Autodesk Inventor part; units mm, degrees
ref_plane "YZ Plane" through (0, 0, 0) normal (1, 0, 0) x (0, 1, 0)
ref_plane "XZ Plane" through (0, 0, 0) normal (0, 1, 0) x (-1, 0, 0)
ref_plane "XY Plane" through (0, 0, 0) normal (0, 0, 1) x (1, 0, 0)
sketch "스케치1" plane through (0, 0, 0) normal (0, 0, 1) x (1, 0, 0)
  line L0 (0, 0) -> (25, 0)
  line L1 (25, 0) -> (25, 16.5)
  line L2 (25, 16.5) -> (0, 16.5)
  line L3 (0, 16.5) -> (0, 0)
  circle A0 centre (23, 14.5) radius 1
  circle A1 centre (2, 14.5) radius 1
  circle A2 centre (2, 2) radius 1
  circle A3 centre (23, 2) radius 1
  circle A4 centre (12.5, 4.5) radius 4.5
  dimension "d0" = 25
  dimension "d1" = 16.5
  dimension "d2" = 2
  dimension "d3" = 2
  dimension "d4" = 2
  dimension "d5" = 2
  dimension "d6" = 2
  dimension "d7" = 2
  dimension "d8" = 2
  dimension "d9" = 2
  dimension "d10" = 2
  dimension "d11" = 2
  dimension "d12" = 2
  dimension "d13" = 2
  dimension "d14" = 12.5
  dimension "d15" = 12.5
  dimension "d18" = 9
  dimension "d19" = 12
  dimension "d20" = 16.5
extrude "돌출1" add sketch "스케치1" along normal blind 2 contours A4 | L3 L2 L1 L0
extrude "돌출2" add sketch "스케치1" against normal blind 160 contours A4
sketch "스케치2" plane through (12.5, 4.5, -160) normal (0, 0, -1) x (-1, 0, 0)
  line L0 (0, 0) -> (10, 0)
  line L1 (10, 0) -> (10, -10)
  line L2 (10, -10) -> (0, -10)
  line L3 (0, -10) -> (0, 0)
  line L4 (10, -10) -> (-10, -10)
  line L5 (-10, -10) -> (-10, 10)
  line L6 (-10, 10) -> (10, 10)
  line L7 (10, 10) -> (10, -10)
  point P0 (12.5, -4.5)
  dimension "d23" = 10
  dimension "d24" = 10
  dimension "d25" = 20
  dimension "d26" = 20
extrude "돌출3" add sketch "스케치2" along normal blind 10
sketch "스케치3" plane through (2.5, -5.5, -160) normal (-1, 0, 0) x (0, 0, 1)
  line L0 (-10, 20) -> (-10, 0)
  line L1 (0, 20) -> (0, 0)
  line L2 (-10, 20) -> (0, 0)
  line L3 (-10, 0) -> (0, 20)
  circle A0 centre (-5, 10) radius 2.5
  line L4 (-5, 12.5) -> (-3.75, 12.1651)
  line L5 (-3.75, 12.1651) -> (-2.8349, 11.25)
  line L6 (-2.8349, 11.25) -> (-2.5, 10)
  line L7 (-2.5, 10) -> (-2.8349, 8.75)
  line L8 (-2.8349, 8.75) -> (-3.75, 7.8349)
  line L9 (-3.75, 7.8349) -> (-5, 7.5)
  line L10 (-5, 7.5) -> (-6.25, 7.8349)
  line L11 (-6.25, 7.8349) -> (-7.1651, 8.75)
  line L12 (-7.1651, 8.75) -> (-7.5, 10)
  line L13 (-7.5, 10) -> (-7.1651, 11.25)
  line L14 (-7.1651, 11.25) -> (-6.25, 12.1651)
  line L15 (-6.25, 12.1651) -> (-5, 12.5)
  point P0 (160, 5.5)
  dimension "d29" = 5
extrude "돌출4" cut sketch "스케치3" against normal blind 15 contours L15 L4 L3 L2 | L2 L3 L10 L11 L12 L13 L14 L15 | L3 L2 L9 L10 | L3 L4 L5 L6 L7 L8 L9 L2
sketch "스케치4" plane through (2.5, 14.5, -160) normal (0, 1, 0) x (1, 0, 0)
  line L0 (17.5, 9) -> (2.5, 9)
  line L1 (2.5, 9) -> (2.5, 7)
  line L2 (2.5, 7) -> (17.5, 7)
  line L3 (17.5, 7) -> (17.5, 9)
  line L4 (0, 10) -> (20, 10)
  line L5 (20, 0) -> (20, 10)
  line L6 (15, 9) -> (5, 9)
  line L7 (5, 9) -> (5, 10)
  line L8 (5, 10) -> (15, 10)
  line L9 (15, 10) -> (15, 9)
  point P0 (-2.5, -160)
  point P1 (15, 9.5)
  point P2 (15, 10)
  point P3 (5, 9)
  dimension "d32" = 15
  dimension "d33" = 2
  dimension "d34" = 1
  dimension "d35" = 2.5
  dimension "d36" = 10
  dimension "d37" = 1
  dimension "d38" = 2.5
extrude "돌출5" cut sketch "스케치4" against normal blind 5
properties part number "camera arm v1_3D 인쇄"
The model under review builds one solid part; all positions refer to its coordinate system, in mm. A direction names the side the tool comes from. Coordinates: 2 decimals unless noted, no trailing zeros. Write each loop counter-clockwise with the first axis right and the second up, starting at its lowest first coordinate (ties: lowest second). Pieces come first, ordered by that corner, then holes. Notation, with made-up numbers: (-35, 9.5) - (-24, 9.5) arc R10 cw to (-24, 15.5) - close; hole circle Ø5 at (-29.75, 67.5). An arc over 180 degrees is marked (long way). Write item = value, one per line.
(1) Mouldability with a two-part tool opening along Z and no side actions: class faces 5 (the face through (12, 9.5, -169)), 6 (the face through (22.5, 4, -165)), 7 (the face through (13, 5, -170)) as pulls with the +Z half, pulls with the -Z half, needs draft (parallel to the pull), parting line crosses it, or undercut.
Result sheet:
face_5 = undercut
face_6 = needs draft
face_7 = pulls with the -Z half
(2) For line 1 (Y direction, x = 2, z = 0.5); line 2 (Z direction, x = 19.75, y = 1); line 3 (Z direction, x = 13.75, y = 4.5), list the stretches that pass through material, from the lowest coordinate up. Write a range as [from, to].
Result sheet:
line_1 = [0, 1], [3, 13.5], [15.5, 16.5]
line_2 = [-170, -160], [0, 2]
line_3 = [-170, -167.5], [-162.5, 2]
(3) Machinability: for faces 1 (the face through (2.5, 7, -164)), 2 (the face through (17.5, 5, -165)), 3 (the face through (17, 7, -160)), 4 (the face through (12, 12, -167)), which of the approach directions +Z, -Z, +X, -X, +Y, -Y give a long, thin tool a straight path to every point of the face, cutting with its end or side? Answer none if there is none.
Result sheet:
face_1 = -Z, -X, +Y, -Y
face_2 = -X
face_3 = none
face_4 = +Y
(4) For P1, Ø8, axis at y = 5.5, z = -163.5, coming from the +X side; P2, Ø12, axis at y = 13.5, z = -142.5, coming from the -X side; P3, Ø1.5, axis at x = 11, z = -169, coming from the +Y side; P4, Ø1.8, axis at x = 2, y = 14.5, coming from the -Z side, all flat-tipped, find the tip position at first contact; note any pin that passes through.
Result sheet:
P1 = 22.5
P2 = 9.15
P3 = 9.5
P4 = -170
(5) Consider section B-B, the plane y = -4. Give the boundary of the cut face in (x, z), then the cut area to 3 significant figures.
Result sheet:
outline = (2.5, -170) - (22.5, -170) - (22.5, -160) - (2.5, -160) - close
area = 200 mm^2
(6) Consider section A-A, the plane z = -38. Give the boundary of the cut face in (x, y).
Result sheet:
outline = circle Ø9 at (12.5, 4.5)
